```python
from build123d import *

# Parameters (mm, degrees)
ESBO_O1_W                = 90
ESBO_O1_H                = 100
ESBO_O1_R                = 1
ESBO_O1_W_2              = 13
ESBO_O1_H_2              = 23.2
RESSALTO_EXTRUS_O1_DEPTH = 25
CORTE_EXTRUS_O1_DEPTH    = 22
ESBO_O4_W                = 90
ESBO_O4_H                = 100
ESBO_O4_R                = 1.6
RESSALTO_EXTRUS_O2_DEPTH = 2.5


with BuildPart() as part:
    # Esboço1 → Ressalto-extrusão1 (new body)
    with BuildSketch(Plane.XY):
        Rectangle(ESBO_O1_W, ESBO_O1_H)
        with Locations((35.5, 19.75)):
            Circle(ESBO_O1_R, mode=Mode.SUBTRACT)
        with Locations((35.5, 47.05)):
            Circle(ESBO_O1_R, mode=Mode.SUBTRACT)
        with Locations(Location((35.5, -47.05, 0), (0, 0, 180))):
            Circle(ESBO_O1_R, mode=Mode.SUBTRACT)
        with Locations(Location((35.5, -19.75, 0), (0, 0, 180))):
            Circle(ESBO_O1_R, mode=Mode.SUBTRACT)
        with Locations((-35.5, -19.75)):
            Circle(ESBO_O1_R, mode=Mode.SUBTRACT)
        with Locations((-35.5, -47.05)):
            Circle(ESBO_O1_R, mode=Mode.SUBTRACT)
        with Locations(Location((-35.5, 47.05, 0), (0, 0, 180))):
            Circle(ESBO_O1_R, mode=Mode.SUBTRACT)
        with Locations(Location((-35.5, 19.75, 0), (0, 0, 180))):
            Circle(ESBO_O1_R, mode=Mode.SUBTRACT)
        with Locations((35.5, 33.4)):
            Rectangle(ESBO_O1_W_2, ESBO_O1_H_2, mode=Mode.SUBTRACT)
        with Locations((35.5, -33.4)):
            Rectangle(ESBO_O1_W_2, ESBO_O1_H_2, mode=Mode.SUBTRACT)
        with Locations((-35.5, -33.4)):
            Rectangle(ESBO_O1_W_2, ESBO_O1_H_2, mode=Mode.SUBTRACT)
        with Locations((-35.5, 33.4)):
            Rectangle(ESBO_O1_W_2, ESBO_O1_H_2, mode=Mode.SUBTRACT)
    extrude(amount=RESSALTO_EXTRUS_O1_DEPTH)

    # Esboço3 → Corte-extrusão1 (cut)
    with BuildSketch(Plane.XY.offset(25)):
        Polygon((-29.5, 47), (29.5, 47), (29.5, 15.8), (42, 15.8), (42, -15.8), (29.5, -15.8), (29.5, -47), (-29.5, -47), (-29.5, -15.8), (-42, -15.8), (-42, 15.8), (-29.5, 15.8), align=None)
    extrude(amount=-CORTE_EXTRUS_O1_DEPTH, mode=Mode.SUBTRACT)

    # Esboço4 → Ressalto-extrusão2 (add)
    with BuildSketch(Plane(origin=(0, 0, 0), x_dir=(-1, 0, 0), z_dir=(0, 0, -1))):
        Rectangle(ESBO_O4_W, ESBO_O4_H)
        with Locations((-35.5, -39.05)):
            Circle(ESBO_O4_R, mode=Mode.SUBTRACT)
        with Locations(Location((-35.5, 39.05, 0), (0, 0, 180))):
            Circle(ESBO_O4_R, mode=Mode.SUBTRACT)
        with Locations((35.5, 39.05)):
            Circle(ESBO_O4_R, mode=Mode.SUBTRACT)
        with Locations(Location((35.5, -39.05, 0), (0, 0, 180))):
            Circle(ESBO_O4_R, mode=Mode.SUBTRACT)
    extrude(amount=-RESSALTO_EXTRUS_O2_DEPTH)


solid = part.part
```
Verification items for the finished model (mm, model axes). A direction names the side the tool comes from. Round coordinates to 2 decimals unless told otherwise and drop trailing zeros. Order: outer loops, then holes, each group sorted by start corner. A loop starts at its lowest first (then second) coordinate and runs counter-clockwise, first axis right, second up. Notation, with made-up numbers: (-6, 3.5) -> (34, 3.5) arc R15 cw to (34, 9.5) -> close; hole circle Ø10 at (50.25, -3). An arc over 180 degrees is marked (long way). Put each result on its own line as item: value. Start each with the question number.
(1) Depth check by flat-ended pin: pin 1 Ø1.6 at (x, y) = (-36, -19.5) entering from +Z. Enter the tip coordinate at first touch or a pass-through.
(2) Tool access check on faces 1 (the face through (-34.23, 38.08, 1.23)), 2 (the face through (36, 15.8, 14)). Record the directions out of +Z, -Z, +X, -X, +Y, -Y that give a thin tool (end or side, any length) a straight path to the whole face; none if there is none.
(3) Section check C-C (z = 14.75). State how many separate pieces and enclosed holes the cut face has, then the cut area to 3 significant figures.
(4) Section check B-B (x = 2). Enter the section's corners in (y, z).
(5) Section check A-A (y = 39.05). Enter the section's corners in (x, z).
(6) Draft check along X on faces 3 (the face through (36, -15.8, 14)), 4 (the face through (-1, 1, 0)), 5 (the face through (-45, -1, 12)), 6 (the face through (35, 45, 14)). Enter one of: +X half, -X half, draft (parallel to the pull), parting line (faces both ways), or undercut.
(7) Material ranges on line 1 along Y through (x, z) = (32.5, 3.5); line 2 along Y through (x, z) = (-35.5, 1.5); line 3 along X through (y, z) = (47.05, 18.5), recorded low to high.
(8) Section check D-D (y = -1.5). Enter the section's corners in (x, z).
Completed:
1. pin 1: stops at z = 25
2. face 1: +Z, -Z
2. face 2: +Z
3. separate pieces: 1
3. enclosed holes: 9
3. area: 1,480 mm2
4. outline: (-50, 0) -> (50, 0) -> (50, 25) -> (47, 25) -> (47, 3) -> (-47, 3) -> (-47, 25) -> (-50, 25) -> close
5. outline: (-45, 0) -> (-37.1, 0) -> (-37.1, 2.5) -> (-42, 2.5) -> (-42, 25) -> (-45, 25) -> close; (-33.9, 0) -> (33.9, 0) -> (33.9, 2.5) -> (29, 2.5) -> (29, 3) -> (-29, 3) -> (-29, 2.5) -> (-33.9, 2.5) -> close; (37.1, 0) -> (45, 0) -> (45, 25) -> (42, 25) -> (42, 2.5) -> (37.1, 2.5) -> close
6. face 3: undercut
6. face 4: draft
6. face 5: -X half
6. face 6: undercut
7. line 1: y = -50 to -45, -21.8 to -15.8, 15.8 to 21.8, 45 to 50
7. line 2: y = -50 to -40.65, -37.45 to 37.45, 40.65 to 50
7. line 3: x = -45 to -36.5, -34.5 to 34.5, 36.5 to 45
8. outline: (-45, 0) -> (45, 0) -> (45, 25) -> (42, 25) -> (42, 3) -> (-42, 3) -> (-42, 25) -> (-45, 25) -> close
